from build123d import *

# Parameters (mm, degrees)
BOX320_W          = 30.2
BOX320_H          = 30.2
BOX320_DEPTH      = 20
CYLINDER816_R     = 24.65
CYLINDER816_DEPTH = 20
CHAMFER006_SIZE   = 0.5
CHAMFER005_SIZE   = 1
CHAMFER007_SIZE   = 0.5


with BuildPart() as krychle320:
    # Box320 → Box320 (new body)
    with BuildSketch(Plane(origin=(-15.1, -15.1, 0), x_dir=(1, 0, 0), z_dir=(0, 0, 1))):
        with Locations((15.1, 15.1)):
            Rectangle(BOX320_W, BOX320_H)
    extrude(amount=BOX320_DEPTH)


with BuildPart() as chamfer007:
    # Cylinder816 → Cylinder816 (new body)
    with BuildSketch(Plane.XY):
        Circle(CYLINDER816_R)
    extrude(amount=CYLINDER816_DEPTH)

    # Cut349: cut Krychle320
    add(krychle320.part, mode=Mode.SUBTRACT)

    # Chamfer006
    chamfer006_edges = [chamfer007.edges().sort_by_distance(p)[0] for p in [
        (0, -15.1, 0),
        (0, 15.1, 0),
    ]]
    chamfer(chamfer006_edges, length=CHAMFER006_SIZE)

    # Chamfer005
    chamfer005_edges = [chamfer007.edges().sort_by_distance(p)[0] for p in [
        (-24.65, 0, 20),
    ]]
    chamfer(chamfer005_edges, length=CHAMFER005_SIZE)

    # Chamfer007
    chamfer007_edges = [chamfer007.edges().sort_by_distance(p)[0] for p in [
        (-24.65, 0, 0),
    ]]
    chamfer(chamfer007_edges, length=CHAMFER007_SIZE)


solid = chamfer007.part
Source: CAD feature listing. Evaluate the final solid. Frame: model axes, mm. A direction names the side the tool comes from. Round coordinates to 2 decimals unless told otherwise and drop trailing zeros. Loops run counter-clockwise (first coordinate to the right, second up) from the corner with the lowest first, then second, coordinate; pieces in that order, holes last.
Q1. Section A-A, the plane x = 0. Return loops of the section in (y, z), plus the area to 4 significant figures.
Q2. Section C-C, the plane z = 15.5. Return loops of the section in (x, y), plus the area to 3 significant figures.
Q3. First-contact query: P1, Ø2, axis at x = 4.5, z = 5, coming from the +Y side; P2, Ø4, axis at x = -12, y = 5, coming from the +Z side; P3, Ø10, axis at x = 10, z = 12, coming from the -Y side; P4, Ø12, axis at y = -13.5, z = 17.5, coming from the +X side. Flat tips, straight axial feed; report the tip coordinate or a pass-through.
Q4. Section B-B, the plane y = 0. Return loops of the section in (x, z).
Q5. Mould query, pull axis Y, two halves, no side actions, for faces 1 (the face through (-5.344, -24.064, 9.62)), 2 (the face through (0, -15.1, 10)), 3 (the face through (-0.3, -15.4, 20)). Classes: pulls with the +Y half, pulls with the -Y half, needs draft (parallel to the pull), parting line crosses it, or undercut.
Q6. Access query for faces 4 (the face through (16, 0, 0)), 5 (the face through (0, 15.1, 10)). Directions: +Z, -Z, +X, -X, +Y, -Y. A direction counts if a zero-diameter tool reaches every point of the face in a straight line with its end or side. Return the directions, or none.
Q7. Ray query, line 1 (X direction, y = 10, z = 17.25); line 2 (Y direction, x = 15, z = 13); line 3 (Y direction, x = -13, z = 16.75). Return the intervals inside material, ascending.
Solutions:
1. outline: (-24.65, 0.5) - (-24.15, 0) - (-15.6, 0) - (-15.1, 0.5) - (-15.1, 20) - (-23.65, 20) - (-24.65, 19) - close; (15.1, 0.5) - (15.6, 0) - (24.15, 0) - (24.65, 0.5) - (24.65, 19) - (23.65, 20) - (15.1, 20) - close
1. area: 380.5 mm2
2. outline: circle Ø49.3 at (0, 0); hole (-15.1, -15.1) - (15.1, -15.1) - (15.1, 15.1) - (-15.1, 15.1) - close
2. area: 997 mm2
3. P1: stops at y = 24.4
3. P2: passes through
3. P3: stops at y = -24.14
3. P4: stops at x = 23.48
4. outline: (-24.65, 0.5) - (-24.15, 0) - (-15.1, 0) - (-15.1, 20) - (-23.65, 20) - (-24.65, 19) - close; (15.1, 0) - (24.15, 0) - (24.65, 0.5) - (24.65, 19) - (23.65, 20) - (15.1, 20) - close
5. face 1: parting line crosses it
5. face 2: undercut
5. face 3: needs draft
6. face 4: -Z, +X, -X, +Y, -Y
6. face 5: +Z, -Z
7. line 1: x = -22.53 to -15.1, 15.1 to 22.53
7. line 2: y = -19.56 to -15.1, 15.1 to 19.56
7. line 3: y = -20.94 to -15.1, 15.1 to 20.94
